Work out the finished part from the listing and answer in its coordinate system (mm). A direction names the side the tool comes from. Give positions to 0.01 mm unless a question says otherwise; leave off trailing zeros. Loops run counter-clockwise (first coordinate to the right, second up) from the corner with the lowest first, then second, coordinate; pieces in that order, holes last. Notation, with made-up numbers: M 54,6 L 84,6 A19 ccw 84,28 Z; hole C -35,31.25 d8. An arc over 180 degrees is marked long. Write item = value, one per line. Start each with the question number.
1. The mould has two halves that part along Z. Classify faces 3 (the face through (-3.66, 22.01, -2.8)), 4 (the face through (3.415, 21.438, -1.416)): released by +Z, released by -Z, zero draft, split by the parting line, or undercut.
2. Section B-B on y = 5 is taken. Determine the outline of the cut face in (x, z), plus the area to 3 significant figures.
3. Consider L1, parallel to X at y = 7.25, z = 0; L2, parallel to Z at x = 0, y = 23. Determine where each line is inside the solid, lowest interval first. Write a range as [from, to].
4. Flat-ended cylindrical pins translate along their axes: pin 1 Ø1 at (x, z) = (0, 2.5) entering from +Y; pin 2 Ø1.5 at (y, z) = (24, -3) entering from -X. Find the tip coordinate at first contact, or state that the pin passes through.
5. For faces 1 (the face through (-0.458, 3.803, 2.064)), 2 (the face through (-2, 9, 0)), determine the directions among +Z, -Z, +X, -X, +Y, -Y from which every point of the face is accessible in a straight line to the end or side of a thin tool.
6. Section A-A on z = 0 is taken. Determine the outline of the cut face in (x, y) (1 decimal).
7. Section C-C on y = 29 is taken. Determine the outline of the cut face in (x, z) (1 decimal).
Autodesk Inventor part; units mm, degrees
ref_plane "YZ Plane" through (0, 0, 0) normal (1, 0, 0) x (0, 1, 0)
ref_plane "XZ Plane" through (0, 0, 0) normal (0, 1, 0) x (-1, 0, 0)
ref_plane "XY Plane" through (0, 0, 0) normal (0, 0, 1) x (1, 0, 0)
sketch "Sketch1" plane through (0, 0, 0) normal (0, 0, 1) x (1, 0, 0)
  line L0 (0, 0) -> (2, 0)
  line L1 (2.225, 7.5) -> (2, 0)
  line L2 (2, 0) -> (1.5, 0)
  line L3 (1.5, 0) -> (1.5, 8.5)
  line L4 (2, 0) -> (1.5, 0)
  line L5 (0.1075, 35.8962) -> (4.6075, 35.8962) construction
  line L6 (3.6973, 32.4828) -> (4.6075, 35.8962)
  line L7 (3.6973, 32.4828) -> (28.4522, 32.4828) construction
  line L8 (1.5, 8.5) -> (3.6973, 10.6973)
  line L9 (1.5, 8.5) -> (4.6075, 8.5) construction
  line L10 (4.6075, 35.8962) -> (4.6075, 8.5)
  line L11 (2.225, 7.5) -> (4.6075, 8.5)
  line L12 (3.6973, 32.4828) -> (3.6973, 10.6973)
  line L13 (2, 0) -> (1.5, 0)
  line L14 (1.5, 0) -> (2, 0)
  line L15 (0, 0) -> (0, 42.8273)
  dimension "d0" = 2
  dimension "d6" = 8.5
  dimension "d20" = 45
revolve "Revolution1" add sketch "Sketch1" angle 360 about axis through (0, 0, 0) along (0, 1, 0)
properties part number "Pipet to Needle"
Verdict:
q1.face_3 = split by the parting line
q1.face_4 = undercut
q2.outline = C 0,0 d4.3; hole C 0,0 d3
q2.area = 7.45 mm2
q3.L1 = [-2.22, -1.5], [1.5, 2.22]
q3.L2 = [-4.61, -3.7], [3.7, 4.61]
q4.pin_1 = 10
q4.pin_2 = -4.02
q5.face_1 = -Y
q5.face_2 = +Y
q6.outline = M -4.6,8.5 L -2.2,7.5 L -2,0 L -1.5,0 L -1.5,8.5 L -3.7,10.7 L -3.7,32.5 L -4.6,35.9 Z; M 1.5,0 L 2,0 L 2.2,7.5 L 4.6,8.5 L 4.6,35.9 L 3.7,32.5 L 3.7,10.7 L 1.5,8.5 Z
q7.outline = C 0,0 d9.2; hole C 0,0 d7.4
